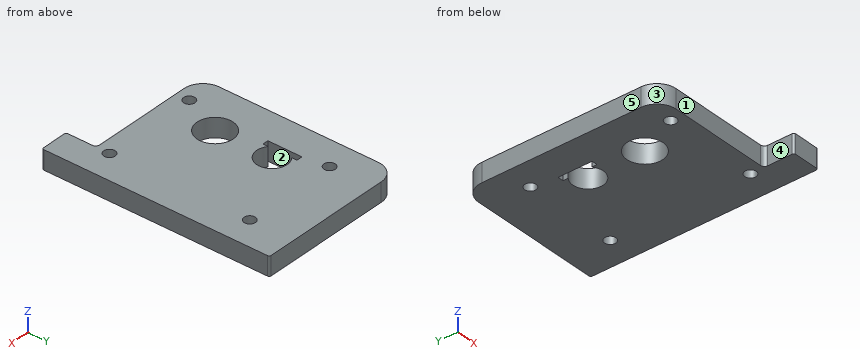
```python
from build123d import *

# Parameters (mm, degrees)
SKETCH_R    = 9.5
SKETCH_R_2  = 3
PAD_DEPTH   = 10
FILLET_R    = 10
FILLET001_R = 2
FILLET002_R = 1


with BuildPart() as part:
    # Sketch → Pad (new body)
    with BuildSketch(Plane.XY):
        Polygon((-25, 45), (55, 45), (55, -75), (40, -75), (40, -59), (-25, -59), align=None)
        with Locations((0, -30)):
            Circle(SKETCH_R, mode=Mode.SUBTRACT)
        with Locations((-10, -52)):
            Circle(SKETCH_R_2, mode=Mode.SUBTRACT)
        with Locations((40, -52)):
            Circle(SKETCH_R_2, mode=Mode.SUBTRACT)
        with Locations((40, 22)):
            Circle(SKETCH_R_2, mode=Mode.SUBTRACT)
        with Locations((-10, 22)):
            Circle(SKETCH_R_2, mode=Mode.SUBTRACT)
        with BuildLine():
            ThreePointArc((-5, -6.244998), (8, 0), (-5, 6.244998))
            Line((-5, 9), (-5, 6.244998))
            Line((-8.125, 9), (-5, 9))
            Line((-8.125, -9), (-8.125, 9))
            Line((-5, -9), (-8.125, -9))
            Line((-5, -6.244998), (-5, -9))
        make_face(mode=Mode.SUBTRACT)
    extrude(amount=PAD_DEPTH)

    # Fillet
    fillet_edges = [part.edges().sort_by_distance(p)[0] for p in [
        (-25, 45, 5),
        (-25, -59, 5),
    ]]
    fillet(fillet_edges, radius=FILLET_R)

    # Fillet001
    fillet001_edges = [part.edges().sort_by_distance(p)[0] for p in [
        (40, -59, 5),
    ]]
    fillet(fillet001_edges, radius=FILLET001_R)

    # Fillet002
    fillet002_edges = [part.edges().sort_by_distance(p)[0] for p in [
        (40, -75, 5),
        (55, -75, 5),
        (55, 45, 5),
    ]]
    fillet(fillet002_edges, radius=FILLET002_R)


solid = part.part
```
Part model, mm, in its own coordinate system. Face numbers are marked on the shaded views. A direction names the side the tool comes from. Give positions to 0.01 mm unless a question says otherwise; leave off trailing zeros. Order: outer loops, then holes, each group sorted by start corner. A loop starts at its lowest first (then second) coordinate and runs counter-clockwise, first axis right, second up. Notation, with made-up numbers: M 62,0 L 121,0 A21 ccw 121,29 Z; hole C -23.5,50.25 d7. An arc over 180 degrees is marked long. Use a Markdown table: item, result. Add a question column.
(1) 3-axis set-ups, long thin cutter, end or side, ignore diameter. For the marked faces 4 and 5: which of +Z, -Z, +X, -X, +Y, -Y reach the whole face in a straight line?
(2) Saw through at D-D, the plane z = 2. Give the cut face in (x, y) (3 decimals).
(3) Probe line 1 along Y through (x, z) = (-10, 7.75); line 2 along Y through (x, z) = (-0.5, 3.25); line 3 along X through (y, z) = (0, 2) (3 decimals). List the from-to ranges inside material, lowest first. Write a range as [from, to].
(4) Saw through at C-C, the plane x = 0. Give the cut face in (y, z), and give its area (3 significant figures).
(5) Saw through at B-B, the plane y = -30. Give the cut face in (x, z).
(6) Drop a flat-ended pin along its axis: P1, Ø5, axis at x = 15.5, z = 6.5, coming from the -Y side. Give the stop position or say it passes through.
(7) Mould opens along X. For the marked faces 1, 2 and 3 say: +X half, -X half, draft (parallel to the pull), parting line (faces both ways), or undercut.
(8) Saw through at A-A, the plane y = 22. Give the cut face in (x, z).
Answer key:
| question | item | result |
|---|---|---|
| 1 | face 4 | +Z, -Z, -X, -Y |
| 1 | face 5 | +Z, -Z, -X, +Y, -Y |
| 2 | outline | M -25,-49 A10 ccw -15,-59 L 38,-59 A2 cw 40,-61 L 40,-74 A1 ccw 41,-75 L 54,-75 A1 ccw 55,-74 L 55,44 A1 ccw 54,45 L -15,45 A10 ccw -25,35 Z; hole C -10,-52 d6; hole C -10,22 d6; hole C 0,-30 d19; hole M -8.125,-9 L -5,-9 L -5,-6.245 A8 ccw long -5,6.245 L -5,9 L -8.125,9 Z; hole C 40,-52 d6; hole C 40,22 d6 |
| 3 | line 1 | [-59, -55], [-49, 19], [25, 45] |
| 3 | line 2 | [-59, -39.49], [-20.51, -7.98], [7.98, 45] |
| 3 | line 3 | [-25, -8.125], [8, 55] |
| 4 | outline | M -59,0 L -39.5,0 L -39.5,10 L -59,10 Z; M -20.5,0 L -8,0 L -8,10 L -20.5,10 Z; M 8,0 L 45,0 L 45,10 L 8,10 Z |
| 4 | area | 690 mm^2 |
| 5 | outline | M -25,0 L -9.5,0 L -9.5,10 L -25,10 Z; M 9.5,0 L 55,0 L 55,10 L 9.5,10 Z |
| 6 | P1 | y = -59 |
| 7 | face 1 | draft |
| 7 | face 2 | undercut |
| 7 | face 3 | -X half |
| 8 | outline | M -25,0 L -13,0 L -13,10 L -25,10 Z; M -7,0 L 37,0 L 37,10 L -7,10 Z; M 43,0 L 55,0 L 55,10 L 43,10 Z |
